```python
from build123d import *

# Parameters (mm, degrees)
CUT_EXTRUDE1_DEPTH = 5.08


with BuildPart() as part:
    # Sketch1 → Revolve3 (revolve)
    with BuildSketch(Plane.XY):
        Polygon((-64.046377149, 7.114962412), (-57.649439031, 7.114962412), (-57.649439031, 6.352962412), (-52.863745559, 6.352962412), (-52.863745559, 4.101714874), (-51.170838104, 4.101714874), (-51.170838104, 6.352962412), (-42.828401085, 6.352962412), (-42.828401085, 7.114962412), (-41.502858565, 7.114962412), (-41.502858565, 7.718234779), (-51.170838104, 7.718234779), (-51.170838104, 9.078659997), (-52.863745559, 9.078659997), (-52.863745559, 7.718234779), (-54.862931861, 7.718234779), (-55.961416497, 7.718234779), (-58.85700077, 7.718234779), (-59.483688957, 7.718234779), (-61.781937161, 7.718234779), (-61.781937161, 7.902812446), (-64.046377149, 7.902812446), align=None)
    revolve(axis=Axis((-52.863745559, 4.101714874, 0), (1, 0, 0)))

    # Sketch4 → Cut-Extrude1 (cut)
    with BuildSketch(Plane.ZY.offset(64.046377149)):
        Polygon((-0.631646969, 7.849963113), (-0.631646969, 8.219502832), (0.464537278, 8.219502832), (0.464537278, 7.849963113), (0.464537278, 0.329109955), (-0.370144054, 0), (-0.631646969, 0.329109955), align=None)
    extrude(amount=-CUT_EXTRUDE1_DEPTH, mode=Mode.SUBTRACT)


solid = part.part
```
Read the model definition and answer for the solid it produces. Units are mm, in the model's axes. A direction names the side the tool comes from. Coordinates: 2 decimals unless noted, no trailing zeros. Write each loop counter-clockwise with the first axis right and the second up, starting at its lowest first coordinate (ties: lowest second). Pieces come first, ordered by that corner, then holes. Notation, with made-up numbers: (73, 67) -> (102, 67) arc R19 ccw to (102, 74) -> close; hole circle Ø8 at (-5.5, 74.5). An arc over 180 degrees is marked (long way). Answer as a JSON object with one key per item and string values.
Q1. The part is cut by section D-D on x = -45.75. Give the vertices of the cut face in (y, z).
The answers:
{"outline": "circle Ø7.23 at (4.1, 0); hole circle Ø4.5 at (4.1, 0)"}
Q2. Flat-ended cylindrical pins translate along their axes: pin 1 Ø0.6 at (x, y) = (-62, 0.5) entering from -Z; pin 2 Ø2 at (x, z) = (-51, 2.5) entering from +Y; pin 3 Ø1 at (x, z) = (-47, 0.5) entering from -Y; pin 4 Ø5 at (y, z) = (4.5, -1) entering from +X. Find the tip coordinate at first contact, or state that the pin passes through.
The answers:
{"pin 1": "stops at z = -1.88", "pin 2": "stops at y = 8.84", "pin 3": "stops at y = 0.49", "pin 4": "stops at x = -41.5"}
Q3. A tool of negligible diameter and unlimited length cuts with its end or side. For faces 1 (the flat face through (-52.864, 4, 0)), 2 (the flat face through (-61.5, 7.5, -0.632)), 3 (the cylindrical face through (-57.39, 7.44, -1.39)), 4 (the flat face through (-51.171, 7, 3)), from which of +Z, -Z, +X, -X, +Y, -Y can it reach the whole face along a straight path? Write none if from no direction.
The answers:
{"face 1": "-X", "face 2": "-X, +Y, -Y", "face 3": "none", "face 4": "+X"}
Q4. Consider line 1 (Y direction, x = -62, z = 0.5); line 2 (X direction, y = 0.75, z = -2.25); line 3 (X direction, y = 6, z = 2.25). Determine where each line is inside the solid, lowest interval first. Write a range as [from, to].
The answers:
{"line 1": "y = [0.33, 1.13], [7.07, 7.87]", "line 2": "x = [-52.86, -51.17]", "line 3": "x = [-57.65, -42.83]"}
Q5. The part is cut by section A-A on z = 0. Give the vertices of the cut face in (x, y), then the cut area to 3 significant figures.
The answers:
{"outline": "(-58.97, 0.49) -> (-52.86, 0.49) -> (-52.86, -0.88) -> (-51.17, -0.88) -> (-51.17, 0.49) -> (-41.5, 0.49) -> (-41.5, 1.09) -> (-42.83, 1.09) -> (-42.83, 1.85) -> (-51.17, 1.85) -> (-51.17, 6.35) -> (-42.83, 6.35) -> (-42.83, 7.11) -> (-41.5, 7.11) -> (-41.5, 7.72) -> (-51.17, 7.72) -> (-51.17, 9.08) -> (-52.86, 9.08) -> (-52.86, 7.72) -> (-58.97, 7.72) -> (-58.97, 7.11) -> (-57.65, 7.11) -> (-57.65, 6.35) -> (-52.86, 6.35) -> (-52.86, 1.85) -> (-57.65, 1.85) -> (-57.65, 1.09) -> (-58.97, 1.09) -> close", "area": "55.9 mm2"}
Q6. Determine the mould class of faces 5 (the cylindrical face through (-46.4, 3.32, -3.53)), 6 (the cylindrical face through (-60.803, 6.976, 0.905)), 7 (the flat face through (-64.046, 3.8, 3.3)) for opening direction Z: pulls with the +Z half, pulls with the -Z half, needs draft (parallel to the pull), parting line crosses it, or undercut.
The answers:
{"face 5": "parting line crosses it", "face 6": "undercut", "face 7": "needs draft"}
